CAD build for the part. Positions are in the model's coordinates, mm. Give positions to 0.01 mm unless a question says otherwise; leave off trailing zeros. Loops run counter-clockwise (first coordinate to the right, second up) from the corner with the lowest first, then second, coordinate; pieces in that order, holes last.
```python
from build123d import *

# Parameters (mm, degrees)
BOSS_EXTRUDE1_DEPTH            = 2
BOSS_EXTRUDE2_DEPTH            = 1.65
F_2_5_2_5_DIAMETER_HOLE1_D     = 2.5
F_2_5_2_5_DIAMETER_HOLE1_DEPTH = 3.65
FILLET1_R                      = 0.5


with BuildPart() as part:
    # Sketch1 → Boss-Extrude1 (new body)
    with BuildSketch(Plane(origin=(0, -0.825, 0), x_dir=(1, 0, 0), z_dir=(0, 1, 0))):
        with BuildLine():
            Line((42, -11), (42, 11))
            ThreePointArc((42, 11), (38, 15), (34, 11))
            Line((34, 11), (34, -11))
            ThreePointArc((34, -11), (38, -15), (42, -11))
        make_face()
    extrude(amount=-BOSS_EXTRUDE1_DEPTH)

    # Sketch2 → Boss-Extrude2 (add)
    with BuildSketch(Plane(origin=(0, -0.825, 0), x_dir=(-1, 0, 0), z_dir=(0, 1, 0))):
        with BuildLine():
            Line((-35.5, 11), (-35.5, -11))
            ThreePointArc((-35.5, -11), (-38, -13.5), (-40.5, -11))
            Line((-40.5, -11), (-40.5, 11))
            ThreePointArc((-40.5, 11), (-38, 13.5), (-35.5, 11))
        make_face()
    extrude(amount=BOSS_EXTRUDE2_DEPTH)

    # Ø2.5 (2.5) Diameter Hole1
    with Locations(Plane(origin=(0, 0.825, 0), x_dir=(1, 0, 0), z_dir=(0, 1, 0))):
        with Locations((38, -11), (38, 11)):
            Hole(F_2_5_2_5_DIAMETER_HOLE1_D / 2, depth=F_2_5_2_5_DIAMETER_HOLE1_DEPTH)

    # Fillet1
    fillet1_edges = [part.edges().sort_by_distance(p)[0] for p in [
        (38, -0.825, 13.5),
        (40.5, -0.825, 0),
        (38, -0.825, -13.5),
        (35.5, -0.825, 0),
    ]]
    fillet(fillet1_edges, radius=FILLET1_R)


solid = part.part
```
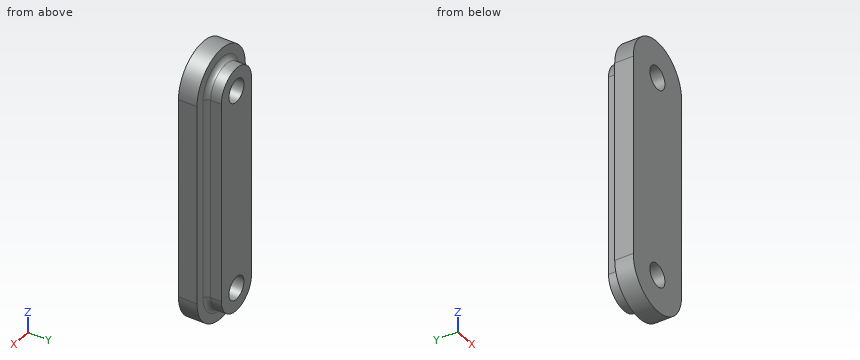
1. Saw through at C-C, the plane z = 9. List the corners of the cut face in (x, y) (3 decimals).
Responses:
outline: (34, -2.825) - (42, -2.825) - (42, -0.825) - (41, -0.825) arc R0.5 cw to (40.5, -0.325) - (40.5, 0.825) - (35.5, 0.825) - (35.5, -0.325) arc R0.5 cw to (35, -0.825) - (34, -0.825) - close
2. Saw through at B-B, the plane x = 38. List the corners of the cut face in (y, z) (3 decimals), and give its area (3 significant figures).
Responses:
outline: (-2.825, -15) - (-0.825, -15) - (-0.825, -14) arc R0.5 cw to (-0.325, -13.5) - (0.825, -13.5) - (0.825, -12.25) - (-2.825, -12.25) - close; (-2.825, -9.75) - (0.825, -9.75) - (0.825, 9.75) - (-2.825, 9.75) - close; (-2.825, 12.25) - (0.825, 12.25) - (0.825, 13.5) - (-0.325, 13.5) arc R0.5 cw to (-0.825, 14) - (-0.825, 15) - (-2.825, 15) - close
area: 86.4 mm2
3. Drop flat-ended pins along their axis: pin 1 (0.9 mm diameter, centred on y = 0.5, z = -2, fed in from +X); pin 2 (0.9 mm diameter, centred on y = 0, z = -5, fed in from -X); pin 3 (1.5 mm diameter, centred on x = 40, y = -2.5, fed in from -Z). Give the stop position or say it passes through.
Responses:
pin 1: stops at x = 40.5
pin 2: stops at x = 35.48
pin 3: stops at z = -14.8
4. Saw through at A-A, the plane y = -2.4. List the corners of the cut face in (x, z), and give its area (3 significant figures).
Responses:
outline: (34, -11) arc R4 ccw to (42, -11) - (42, 11) arc R4 ccw to (34, 11) - close; hole circle Ø2.5 at (38, -11); hole circle Ø2.5 at (38, 11)
area: 216 mm2
5. Saw through at D-D, the plane y = 0.2. List the corners of the cut face in (x, z), and give its area (3 significant figures).
Responses:
outline: (35.5, -11) arc R2.5 ccw to (40.5, -11) - (40.5, 11) arc R2.5 ccw to (35.5, 11) - close; hole circle Ø2.5 at (38, -11); hole circle Ø2.5 at (38, 11)
area: 120 mm2
6. Probe line 1 along Z through (x, y) = (37, 0.3); line 2 along Z through (x, y) = (38.75, -0.15); line 3 along X through (y, z) = (-1.05, -11). List the from-to ranges inside material, lowest first.
Responses:
line 1: z = -13.29 to -11.75, -10.25 to 10.25, 11.75 to 13.29
line 2: z = -13.38 to -12, -10 to 10, 12 to 13.38
line 3: x = 34 to 36.75, 39.25 to 42
